Design review of the part shown in the three views and the two pictorial views. Dimensions are in mm from the part's minimum x, y and z. Give positions to 0.01 mm unless a question says otherwise; leave off trailing zeros. Loops run counter-clockwise (first coordinate to the right, second up) from the corner with the lowest first, then second, coordinate; pieces in that order, holes last.
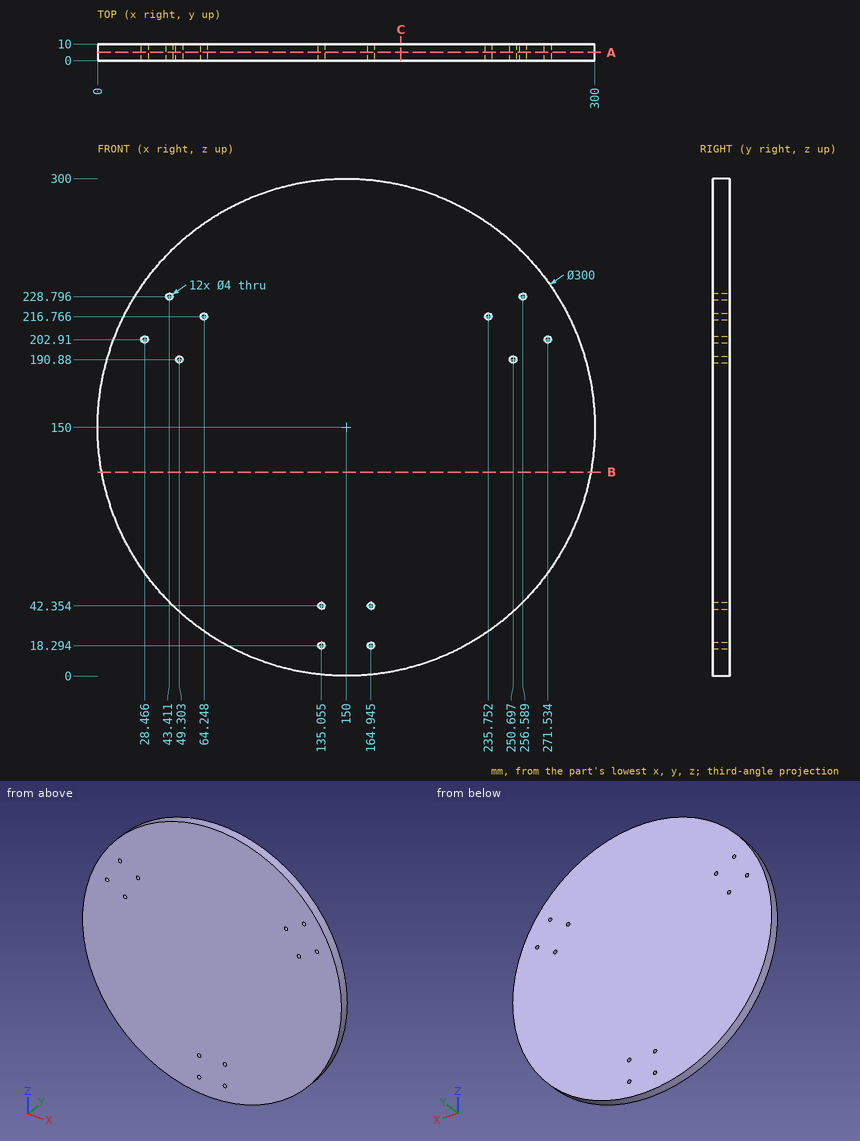
Q1. Consider section A-A on y = 5. Count the separate pieces of the cut face and the enclosed holes in it, plus the area to 3 significant figures.
Answers:
separate pieces: 1
enclosed holes: 12
area: 70,500 mm2
Q2. For pin 1 Ø3 at (y, z) = (2.5, 135) entering from -X, flat-tipped, find the tip position at first contact; note if it passes through.
Answers:
pin 1: stops at x = 0.61
Q3. Consider section C-C on x = 183. Give the boundary of the cut face in (y, z) (1 decimal), plus the area to 3 significant figures.
Answers:
outline: (0, 3.7) - (10, 3.7) - (10, 296.3) - (0, 296.3) - close
area: 2,930 mm2
Q4. For probe 1 along X at (y, z) = (1.5, 216.5) (1 decimal); probe 2 along Z at (x, y) = (135, 1.75) (1 decimal); probe 3 along X at (y, z) = (4.25, 126.5), list the stretches that pass through material, from the lowest coordinate up.
Answers:
probe 1: x = 15.5 to 62.3, 66.2 to 233.8, 237.7 to 284.5
probe 2: z = 0.8 to 16.3, 20.3 to 40.4, 44.4 to 299.2
probe 3: x = 1.85 to 298.15
Q5. Consider section B-B on z = 123. Give the boundary of the cut face in (x, y).
Answers:
outline: (2.45, 0) - (297.55, 0) - (297.55, 10) - (2.45, 10) - close
